Study the drawing (mm; zero at the part's minimum x, y, z) and answer. A direction names the side the tool comes from. Give positions to 0.01 mm unless a question says otherwise; leave off trailing zeros. Loops run counter-clockwise (first coordinate to the right, second up) from the corner with the lowest first, then second, coordinate; pieces in that order, holes last. Notation, with made-up numbers: (86.5, 45.5) - (111.5, 45.5) arc R29 ccw to (111.5, 84.5) - close; hole circle Ø2 at (-29.5, 14.5). An arc over 180 degrees is marked (long way). Write item = value, one per line. Start each with the question number.
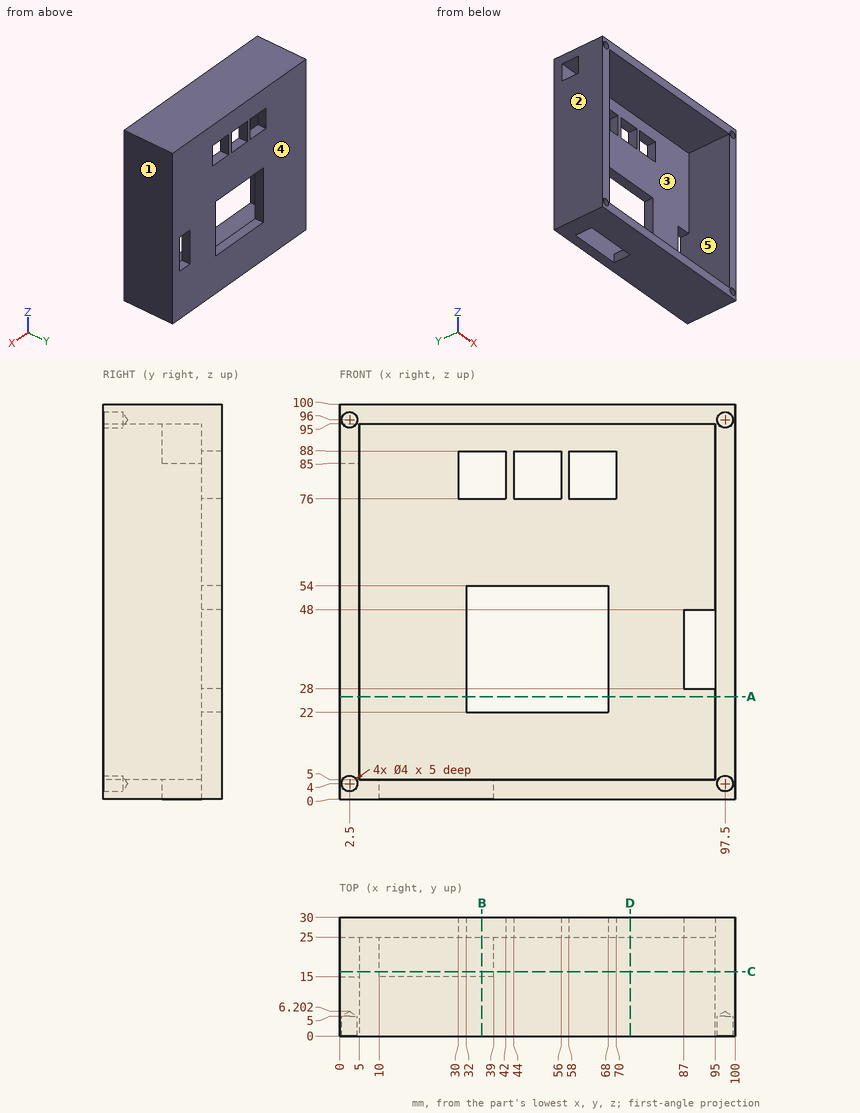
1. A cutting plane is placed at A-A on z = 26. Give the vertices of the cut face in (x, y).
2. A cutting plane is placed at B-B on x = 36. Give the vertices of the cut face in (y, z).
3. Consider line 1 along Z through (x, y) = (2.5, 2); line 2 along X through (y, z) = (1.6, 96); line 3 along X through (y, z) = (18.5, 20). Determine where each line is inside the solid, lowest interval first. Write a range as [from, to].
4. A cutting plane is placed at D-D on x = 73.5. Give the vertices of the cut face in (y, z).
5. Given P1, Ø3.5, axis at x = 2.5, z = 4, coming from the -Y side, flat-ended and moving along its own axis, determine where the tip first touches the part or whether it passes through.
6. For a pull along X with two mould halves and no side action, classify the marked faces 1, 2 and 3 as released by +X, released by -X, zero draft, split by the parting line, or undercut.
7. A cutting plane is placed at C-C on y = 16.25. Give the vertices of the cut face in (x, z), and give its area (4 significant figures).
8. A tool of negligible diameter and unlimited length cuts with its end or side. For the marked faces 4 and 5, from which of +Z, -Z, +X, -X, +Y, -Y can it reach the whole face along a straight path? Write none if from no direction.
Reply:
q1.outline = (0, 0) - (5, 0) - (5, 25) - (32, 25) - (32, 30) - (0, 30) - close; (68, 25) - (95, 25) - (95, 0) - (100, 0) - (100, 30) - (68, 30) - close
q2.outline = (0, 0) - (15, 0) - (15, 5) - (0, 5) - close; (0, 95) - (25, 95) - (25, 88) - (30, 88) - (30, 100) - (0, 100) - close; (25, 0) - (30, 0) - (30, 22) - (25, 22) - close; (25, 54) - (30, 54) - (30, 76) - (25, 76) - close
q3.line_1 = [0, 2], [6, 94], [98, 100]
q3.line_2 = [0, 0.5], [4.5, 95.5], [99.5, 100]
q3.line_3 = [0, 5], [95, 100]
q4.outline = (0, 0) - (30, 0) - (30, 100) - (0, 100) - (0, 95) - (25, 95) - (25, 5) - (0, 5) - close
q5.P1 = 5.15
q6.face_1 = released by +X
q6.face_2 = released by -X
q6.face_3 = undercut
q7.outline = (0, 0) - (10, 0) - (10, 5) - (5, 5) - (5, 85) - (0, 85) - close; (0, 95) - (95, 95) - (95, 5) - (39, 5) - (39, 0) - (100, 0) - (100, 100) - (0, 100) - close
q7.area = 1,705 mm^2
q8.face_4 = +Z, -Z, +X, -X, +Y
q8.face_5 = -Y
